Design review of the part built by this model. Coordinates are the model's own, in mm. Round coordinates to 2 decimals unless told otherwise and drop trailing zeros. Loops run counter-clockwise (first coordinate to the right, second up) from the corner with the lowest first, then second, coordinate; pieces in that order, holes last. Notation, with made-up numbers: M 71,12 L 84,12 A18 cw 84,35 Z; hole C -24.5,28 d8. An arc over 180 degrees is marked long. Use a Markdown table: item, result.
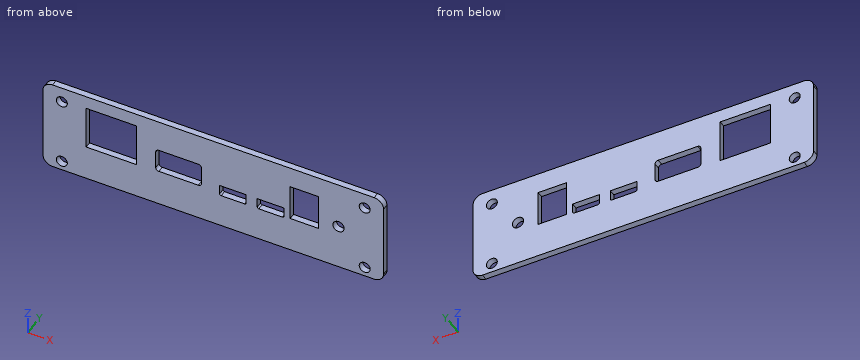
from build123d import *

# Parameters (mm, degrees)
SKETCH1_W           = 108.5
SKETCH1_H           = 29.5
BOSS_EXTRUDE1_DEPTH = 2
SKETCH2_R           = 1.75
CUT_EXTRUDE1_DEPTH  = 113.456658318
FILLET1_R           = 3
SKETCH5_R           = 1.8
SKETCH5_W           = 16
SKETCH5_H           = 14
SKETCH5_W_2         = 14.6
SKETCH5_H_2         = 7.6
SKETCH5_W_3         = 9
SKETCH5_H_3         = 11.5
CUT_EXTRUDE2_DEPTH  = 113.456658318
FILLET2_R           = 1
FILLET3_R           = 0.5


with BuildPart() as part:
    # Sketch1 → Boss-Extrude1 (new body)
    with BuildSketch(Plane(origin=(0, 0, 0), x_dir=(1, 0, 0), z_dir=(0, 1, 0))):
        with Locations((54.25, 14.75)):
            Rectangle(SKETCH1_W, SKETCH1_H)
    extrude(amount=BOSS_EXTRUDE1_DEPTH)

    # Sketch2 → Cut-Extrude1 (cut, through all)
    with BuildSketch(Plane(origin=(0, 2, 0), x_dir=(1, 0, 0), z_dir=(0, 1, 0))):
        with Locations(Location((6, 26.45, 0), (0, 0, 270))):
            Circle(SKETCH2_R)
        with Locations(Location((6, 4.95, 0), (0, 0, 270))):
            Circle(SKETCH2_R)
        with Locations(Location((102.5, 4.95, 0), (0, 0, 90))):
            Circle(SKETCH2_R)
        with Locations(Location((102.5, 26.45, 0), (0, 0, 90))):
            Circle(SKETCH2_R)
    extrude(amount=-CUT_EXTRUDE1_DEPTH, mode=Mode.SUBTRACT)

    # Fillet1
    fillet1_edges = [part.edges().sort_by_distance(p)[0] for p in [
        (0, 1, -29.5),
        (108.5, 1, -29.5),
        (108.5, 1, 0),
        (0, 1, 0),
    ]]
    fillet(fillet1_edges, radius=FILLET1_R)

    # Sketch5 → Cut-Extrude2 (cut, through all)
    with BuildSketch(Plane(origin=(0, 2, 0), x_dir=(1, 0, 0), z_dir=(0, 1, 0))):
        with Locations(Location((94.15, 15, 0), (0, 0, 270))):
            Circle(SKETCH5_R)
        with Locations((21.75, 11.2)):
            Rectangle(SKETCH5_W, SKETCH5_H)
        with Locations((43.2, 14)):
            Rectangle(SKETCH5_W_2, SKETCH5_H_2)
        Polygon((56.25, 18.2), (56.25, 15.2), (64.75, 15.2), (64.75, 18.2), (64.75, 18.7), (56.25, 18.7), align=None)
        Polygon((68.25, 18.2), (68.25, 15.2), (76.75, 15.2), (76.75, 18.2), (76.75, 18.7), (68.25, 18.7), align=None)
        with Locations((83.25, 12.45)):
            Rectangle(SKETCH5_W_3, SKETCH5_H_3)
    extrude(amount=-CUT_EXTRUDE2_DEPTH, mode=Mode.SUBTRACT)

    # Fillet2
    fillet2_edges = [part.edges().sort_by_distance(p)[0] for p in [
        (50.5, 1, -10.2),
        (35.9, 1, -10.2),
        (35.9, 1, -17.8),
        (50.5, 1, -17.8),
    ]]
    fillet(fillet2_edges, radius=FILLET2_R)

    # Fillet3
    fillet3_edges = [part.edges().sort_by_distance(p)[0] for p in [
        (56.25, 1, -18.7),
        (64.75, 1, -18.7),
        (68.25, 1, -18.7),
        (76.75, 1, -18.7),
    ]]
    fillet(fillet3_edges, radius=FILLET3_R)


solid = part.part
1. Insertion check: pin 1 (12 mm diameter, centred on x = 44, z = -23, fed in from -Y); pin 2 (3 mm diameter, centred on x = 6, z = -26.45, fed in from +Y). Each pin has a flat end and moves straight along its axis. Give the tip position at first contact, or say it passes through.
Check values:
| item | result |
|---|---|
| pin 1 | stops at y = 0 |
| pin 2 | passes through |
2. Wall thickness on line 1 along X through (y, z) = (0.85, -26.45); line 2 along Z through (x, y) = (102.5, 0.7); line 3 along X through (y, z) = (0.3, -15): over which ranges is each line inside the solid? List them lowest first. Write a range as from..to.
Check values:
| item | result |
|---|---|
| line 1 | x = 0..4.25, 7.75..100.75, 104.25..108.5 |
| line 2 | z = -29.5..-28.2, -24.7..-6.7, -3.2..0 |
| line 3 | x = 0..13.75, 29.75..35.9, 50.5..78.75, 87.75..92.35, 95.95..108.5 |
3. Take a section at C-C on x = 72. Give the boundary of the cut face in (y, z).
Check values:
| item | result |
|---|---|
| outline | M 0,-29.5 L 2,-29.5 L 2,-18.7 L 0,-18.7 Z; M 0,-15.2 L 2,-15.2 L 2,0 L 0,0 Z |
4. Take a section at B-B on x = 94.15. Give the boundary of the cut face in (y, z).
Check values:
| item | result |
|---|---|
| outline | M 0,-29.5 L 2,-29.5 L 2,-16.8 L 0,-16.8 Z; M 0,-13.2 L 2,-13.2 L 2,0 L 0,0 Z |
5. Take a section at D-D on y = 0.35. Count the separate pieces of the cut face and the enclosed holes in it, and give its area (3 significant figures).
Check values:
| item | result |
|---|---|
| separate pieces | 1 |
| enclosed holes | 10 |
| area | 2,650 mm² |
6. Take a section at A-A on x = 6. Give the boundary of the cut face in (y, z), and give its area (3 significant figures).
Check values:
| item | result |
|---|---|
| outline | M 0,-29.5 L 2,-29.5 L 2,-28.2 L 0,-28.2 Z; M 0,-24.7 L 2,-24.7 L 2,-6.7 L 0,-6.7 Z; M 0,-3.2 L 2,-3.2 L 2,0 L 0,0 Z |
| area | 45.0 mm² |
